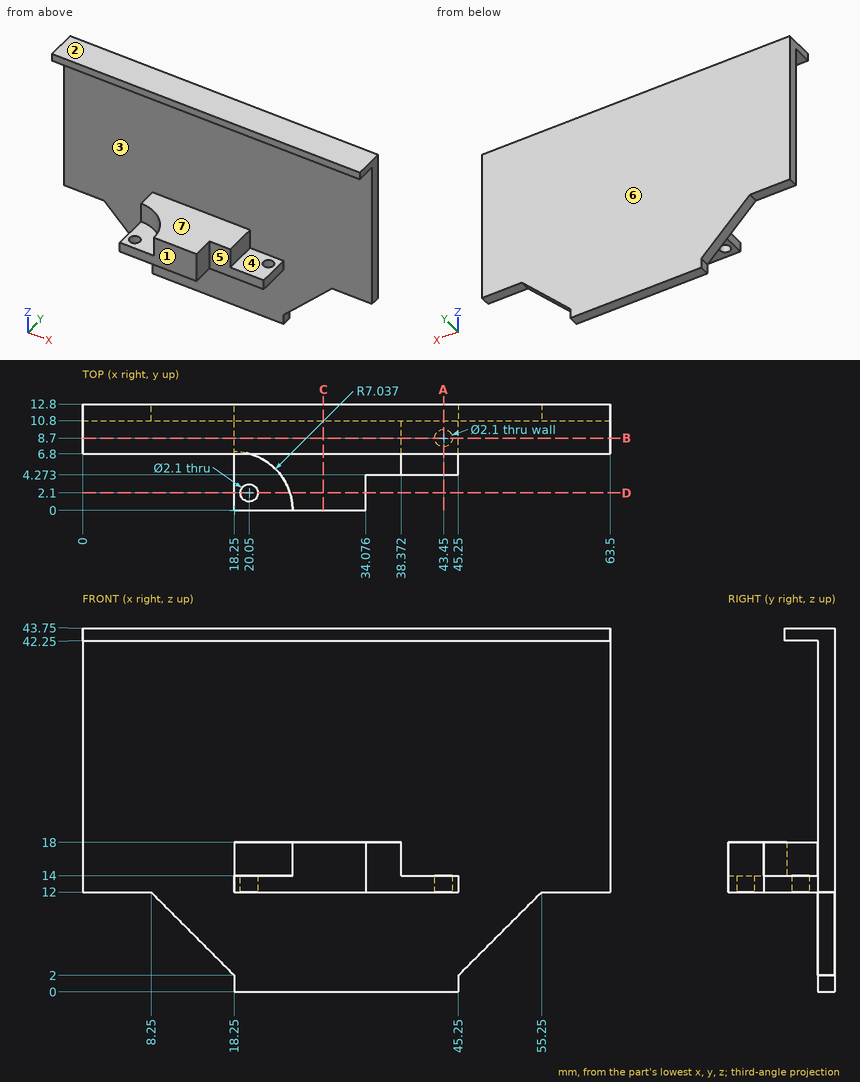
Study the drawing (mm; zero at the part's minimum x, y, z) and answer. A direction names the side the tool comes from. Coordinates: 2 decimals unless noted, no trailing zeros. Write each loop counter-clockwise with the first axis right and the second up, starting at its lowest first coordinate (ties: lowest second). Pieces come first, ordered by that corner, then holes. Notation, with made-up numbers: M 16.5,3.25 L 62.5,3.25 A25 cw 62.5,28.25 Z; hole C 67.25,-27 d4. An arc over 180 degrees is marked long. Use a Markdown table: item, result. Add a question column.
1. Section C-C (x = 29) is taken. Give the vertices of the cut face in (y, z), plus the area to 3 significant figures.
2. Straight lines are drawn through the part: line 1 along Y through (x, z) = (20.05, 12.55); line 2 along Y through (x, z) = (43.45, 12.95); line 3 along Z through (x, y) = (16.5, 10.25). For each, find the intervals that lie inside material, in ascending order. Write a range as [from, to].
3. Section D-D (y = 2.1) is taken. Give the vertices of the cut face in (x, z), plus the area to 3 significant figures.
4. For a pull along Z with two mould halves and no side action, classify the marked faces 1, 2, 3 and 4 as +Z half, -Z half, draft (parallel to the pull), parting line (faces both ways), or undercut.
5. Which of the six approach directions +Z, -Z, +X, -X, +Y, -Y give full straight-line access (tool end or side, diameter ignored) to the marked faces 5, 6 and 7?
6. Section B-B (y = 8.7) is taken. Give the vertices of the cut face in (x, z).
7. Section A-A (x = 43.45) is taken. Give the vertices of the cut face in (y, z), plus the area to 3 significant figures.
8. Given P1, Ø4.5, axis at x = 18, y = 9.5, coming from the -Z side; P2, Ø4.5, axis at y = 2.5, z = 16.5, coming from the +X side; P3, Ø1, axis at x = 58.5, y = 11.5, coming from the -Z side; P4, Ø1.6, axis at y = 12, z = 1, coming from the -X side, each flat-ended and moving along its own axis, determine where each tip first touches the part or whether it passes through.
Data:
| question | item | result |
|---|---|---|
| 1 | outline | M 0,12 L 10.8,12 L 10.8,0 L 12.8,0 L 12.8,43.75 L 6.8,43.75 L 6.8,42.25 L 10.8,42.25 L 10.8,18 L 0,18 Z |
| 1 | area | 158 mm2 |
| 2 | line 1 | y = [0, 1.05], [3.15, 12.8] |
| 2 | line 2 | y = [4.27, 7.65], [9.75, 12.8] |
| 2 | line 3 | z = [42.25, 43.75] |
| 3 | outline | M 18.25,12 L 19,12 L 19,14 L 18.25,14 Z; M 21.1,12 L 34.08,12 L 34.08,18 L 24.97,18 L 24.97,14 L 21.1,14 Z |
| 3 | area | 63.9 mm2 |
| 4 | face 1 | draft |
| 4 | face 2 | +Z half |
| 4 | face 3 | undercut |
| 4 | face 4 | undercut |
| 5 | face 5 | +Z, -Z, +X, -Y |
| 5 | face 6 | +Z, -Z, +X, -X, +Y |
| 5 | face 7 | +X, -X, -Y |
| 6 | outline | M 0,42.25 L 63.5,42.25 L 63.5,43.75 L 0,43.75 Z; M 18.25,12 L 42.4,12 L 42.4,14 L 38.37,14 L 38.37,18 L 18.25,18 Z; M 44.5,12 L 45.25,12 L 45.25,14 L 44.5,14 Z |
| 7 | outline | M 4.27,12 L 7.65,12 L 7.65,14 L 4.27,14 Z; M 6.8,42.25 L 10.8,42.25 L 10.8,14 L 9.75,14 L 9.75,12 L 10.8,12 L 10.8,0 L 12.8,0 L 12.8,43.75 L 6.8,43.75 Z |
| 7 | area | 102 mm2 |
| 8 | P1 | stops at z = 0 |
| 8 | P2 | stops at x = 38.37 |
| 8 | P3 | stops at z = 12 |
| 8 | P4 | stops at x = 18.25 |
